Source: three-view drawing plus pictorial views. Frame: mm from the lowest corner of the part. A direction names the side the tool comes from. Give positions to 0.01 mm unless a question says otherwise; leave off trailing zeros. Write each loop counter-clockwise with the first axis right and the second up, starting at its lowest first coordinate (ties: lowest second). Pieces come first, ordered by that corner, then holes. Notation, with made-up numbers: (17, -35.5) - (21, -35.5) arc R22 cw to (21, -13.5) - close; hole circle Ø2 at (65, -6). An arc over 180 degrees is marked (long way). One line per question, with ' | ' between items. Start each with the question number.
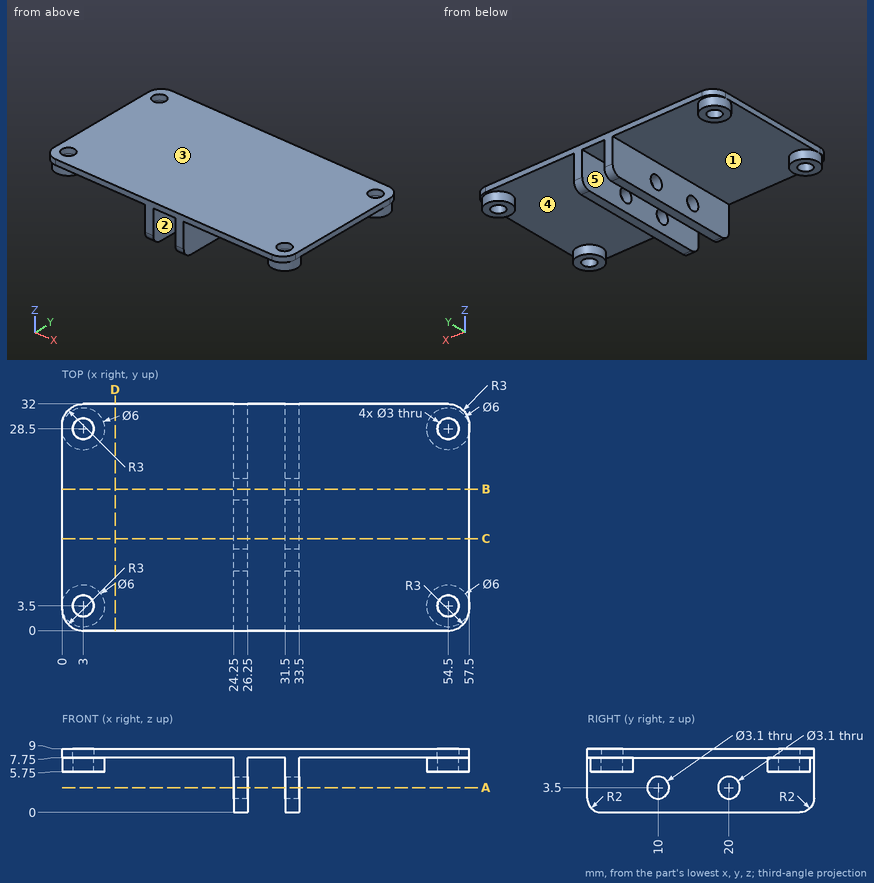
1) Section C-C, the plane y = 13. Output: boundary loops of the cut face in (x, z), plus the area to 3 significant figures.
2) Section A-A, the plane z = 3.5. Output: boundary loops of the cut face in (x, y).
3) Line query: L1, parallel to Y at x = 54.5, z = 7.35; L2, parallel to Y at x = 32.95, z = 3.5; L3, parallel to X at y = 8.5, z = 2. Output: solid intervals per line, ascending.
4) First-contact query: pin 1 Ø1.5 at (x, y) = (44.5, 11) entering from -Z; pin 2 Ø2.5 at (y, z) = (11, 3) entering from -X; pin 3 Ø3 at (x, y) = (53, 28.5) entering from -Z. Flat tips, straight axial feed; report the tip coordinate or a pass-through.
5) Reachability of the marked faces 3, 4 and 5 from +Z, -Z, +X, -X, +Y, -Y: full face, straight path, thin tool, end or side. Return the list, or none.
6) Pull-direction query (Y, two-part tool) for the marked faces 1 and 2; classes: +Y half, -Y half, draft (parallel to the pull), parting line (faces both ways), or undercut.
7) Section D-D, the plane x = 7.5. Output: boundary loops of the cut face in (y, z).
8) Section B-B, the plane y = 20. Output: boundary loops of the cut face in (x, z), plus the area to 3 significant figures.
Answer key:
1) outline: (0, 7.75) - (24.25, 7.75) - (24.25, 0) - (26.25, 0) - (26.25, 7.75) - (31.5, 7.75) - (31.5, 0) - (33.5, 0) - (33.5, 7.75) - (57.5, 7.75) - (57.5, 9) - (0, 9) - close | area: 103 mm^2
2) outline: (24.25, 0) - (26.25, 0) - (26.25, 8.45) - (24.25, 8.45) - close; (24.25, 11.55) - (26.25, 11.55) - (26.25, 18.45) - (24.25, 18.45) - close; (24.25, 21.55) - (26.25, 21.55) - (26.25, 32) - (24.25, 32) - close; (31.5, 0) - (33.5, 0) - (33.5, 8.45) - (31.5, 8.45) - close; (31.5, 11.55) - (33.5, 11.55) - (33.5, 18.45) - (31.5, 18.45) - close; (31.5, 21.55) - (33.5, 21.55) - (33.5, 32) - (31.5, 32) - close
3) L1: 0.5 to 2, 5 to 6.5, 25.5 to 27, 30 to 31.5 | L2: 0 to 8.45, 11.55 to 18.45, 21.55 to 32 | L3: 24.25 to 26.25, 31.5 to 33.5
4) pin 1: z = 7.75 | pin 2: x = 24.25 | pin 3: z = 5.75
5) face 3: +Z, +X, -X, +Y, -Y | face 4: -Z | face 5: -Z, +Y, -Y
6) face 1: undercut | face 2: draft
7) outline: (0, 7.75) - (32, 7.75) - (32, 9) - (0, 9) - close
8) outline: (0, 7.75) - (24.25, 7.75) - (24.25, 5.05) - (26.25, 5.05) - (26.25, 7.75) - (31.5, 7.75) - (31.5, 5.05) - (33.5, 5.05) - (33.5, 7.75) - (57.5, 7.75) - (57.5, 9) - (0, 9) - close; (24.25, 0) - (26.25, 0) - (26.25, 1.95) - (24.25, 1.95) - close; (31.5, 0) - (33.5, 0) - (33.5, 1.95) - (31.5, 1.95) - close | area: 90.5 mm^2
